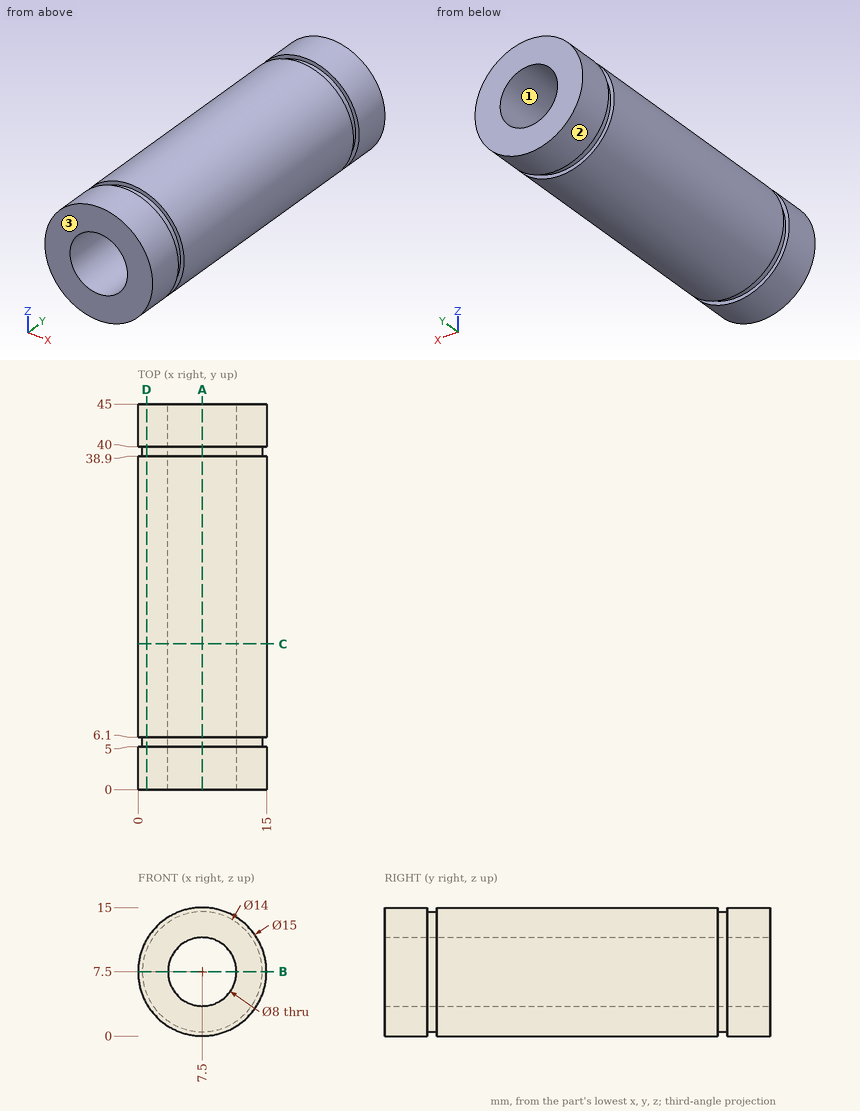
Could you check a few things on this drawing? It's one solid part, dimensions in mm from its lowest x, y, z. Coordinates: 2 decimals unless noted, no trailing zeros. Write each loop counter-clockwise with the first axis right and the second up, starting at its lowest first coordinate (ties: lowest second). Pieces come first, ordered by that corner, then holes. Notation, with made-up numbers: (18, 46) - (27, 46) arc R23 cw to (27, 84) - close; hole circle Ø4 at (5, 51.5). An arc over 180 degrees is marked (long way). Put each result on its own line as item: value. Start each with the question number.
Q1. Thinking about a two-plate mould opening in X: for the marked faces 1, 2 and 3, which applies, pulls with the +X half, pulls with the -X half, needs draft (parallel to the pull), parting line crosses it, or undercut?
Q2. I want a section at B-B on z = 7.5. Write out the boundary of the cut face in (x, y), plus the area to 3 significant figures.
Q3. I want a section at A-A on x = 7.5. Write out the boundary of the cut face in (y, z), plus the area to 3 significant figures.
Q4. I'm going to push flat-ended pins straight in: P1, Ø1.5, axis at x = 12.5, y = 33.5, coming from the +Z side; P2, Ø2, axis at y = 21.5, z = 4.5, coming from the -X side; P3, Ø2, axis at x = 4.5, y = 35.5, coming from the -Z side. Where does each tip first touch, or does it pass through?
Q5. Please list where these lines run through material, in increasing order: L1, parallel to Y at x = 4, z = 1; L2, parallel to Z at x = 7.5, y = 27.5; L3, parallel to X at y = 12, z = 10.
Q6. I want a section at D-D on x = 1. Write out the boundary of the cut face in (y, z), plus the area to 3 significant figures.
Q7. I want a section at C-C on y = 17. Write out the boundary of the cut face in (x, z), plus the area to 3 significant figures.
Checks:
1. face 1: undercut
1. face 2: parting line crosses it
1. face 3: needs draft
2. outline: (0, 0) - (3.5, 0) - (3.5, 45) - (0, 45) - (0, 40) - (0.5, 40) - (0.5, 38.9) - (0, 38.9) - (0, 6.1) - (0.5, 6.1) - (0.5, 5) - (0, 5) - close; (11.5, 0) - (15, 0) - (15, 5) - (14.5, 5) - (14.5, 6.1) - (15, 6.1) - (15, 38.9) - (14.5, 38.9) - (14.5, 40) - (15, 40) - (15, 45) - (11.5, 45) - close
2. area: 313 mm²
3. outline: (0, 0) - (5, 0) - (5, 0.5) - (6.1, 0.5) - (6.1, 0) - (38.9, 0) - (38.9, 0.5) - (40, 0.5) - (40, 0) - (45, 0) - (45, 3.5) - (0, 3.5) - close; (0, 11.5) - (45, 11.5) - (45, 15) - (40, 15) - (40, 14.5) - (38.9, 14.5) - (38.9, 15) - (6.1, 15) - (6.1, 14.5) - (5, 14.5) - (5, 15) - (0, 15) - close
3. area: 313 mm²
4. P1: z = 13.68
4. P2: x = 0.27
4. P3: z = 0.27
5. L1: 0 to 5, 6.1 to 38.9, 40 to 45
5. L2: 0 to 3.5, 11.5 to 15
5. L3: 0.43 to 4.38, 10.62 to 14.57
6. outline: (0, 3.76) - (5, 3.76) - (5, 4.9) - (6.1, 4.9) - (6.1, 3.76) - (38.9, 3.76) - (38.9, 4.9) - (40, 4.9) - (40, 3.76) - (45, 3.76) - (45, 11.24) - (40, 11.24) - (40, 10.1) - (38.9, 10.1) - (38.9, 11.24) - (6.1, 11.24) - (6.1, 10.1) - (5, 10.1) - (5, 11.24) - (0, 11.24) - close
6. area: 332 mm²
7. outline: circle Ø15 at (7.5, 7.5); hole circle Ø8 at (7.5, 7.5)
7. area: 126 mm²
